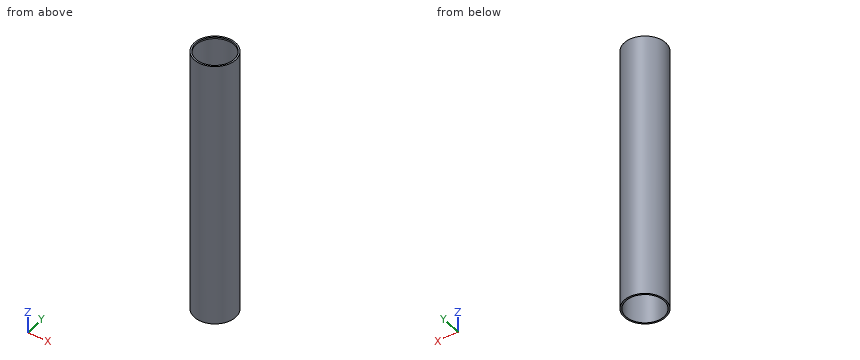
from build123d import *

# Parameters (mm, degrees)
F0_R     = 50.8
F1_DEPTH = 660.4
F2_T     = -3.81
F3_R     = 46.99
F4_DEPTH = 660.401


with BuildPart() as f1:
    # F0 (on Top) → F1 (new body)
    with BuildSketch(Plane.XY):
        Circle(F0_R)
    extrude(amount=F1_DEPTH)

    # F2
    f2_openings = [f1.faces().sort_by_distance(p)[0] for p in [
        (0, 0, 0),
    ]]
    offset(amount=F2_T, openings=f2_openings)

    # F3 (on face) → F4 (cut, through all)
    with BuildSketch(Plane(origin=(0, 0, 0), x_dir=(1, 0, 0), z_dir=(0, 0, -1))):
        Circle(F3_R)
    extrude(amount=-F4_DEPTH, mode=Mode.SUBTRACT)


solid = f1.part
Source: CAD feature listing. Evaluate the final solid. Frame: model axes, mm. Round coordinates to 2 decimals unless told otherwise and drop trailing zeros. Order: outer loops, then holes, each group sorted by start corner. A loop starts at its lowest first (then second) coordinate and runs counter-clockwise, first axis right, second up. Notation, with made-up numbers: (-26.5, 40) -> (14.5, 40) arc R27 cw to (14.5, 62) -> close; hole circle Ø5 at (-37.5, 33). An arc over 180 degrees is marked (long way). Answer as CSV lines item,"result".
Item 1: Section A-A, the plane x = 0. Return loops of the section in (y, z).
A:
outline,"(-50.8, 0) -> (-46.99, 0) -> (-46.99, 660.4) -> (-50.8, 660.4) -> close; (46.99, 0) -> (50.8, 0) -> (50.8, 660.4) -> (46.99, 660.4) -> close"
Item 2: Pin query (flat end, axial travel): pin 1 Ø2 at (x, z) = (-27.5, 289) entering from -Y; pin 2 Ø3 at (x, z) = (-34, 453.5) entering from -Y; pin 3 Ø1 at (x, y) = (-23.5, -40) entering from +Z; pin 4 Ø3 at (y, z) = (9, 199) entering from -X. Return the tip coordinate at first contact, or that it passes through.
A:
pin 1,"y = -43.34"
pin 2,"y = -39.04"
pin 3,"through"
pin 4,"x = -50.24"
Item 3: Section C-C, the plane z = 475. Return loops of the section in (x, y), plus the area to 3 significant figures.
A:
outline,"circle Ø101.6 at (0, 0); hole circle Ø93.98 at (0, 0)"
area,"1,170 mm²"
Item 4: Line query: L1, parallel to Y at x = 0, z = 350.5; L2, parallel to X at y = 31, z = 75. Output: solid intervals per line, ascending.
A:
L1,"-50.8 to -46.99, 46.99 to 50.8"
L2,"-40.24 to -35.31, 35.31 to 40.24"
